from build123d import *

# Parameters (mm, degrees)
SKETCH1_R           = 32.5
BOSS_EXTRUDE1_DEPTH = 230
SKETCH2_R           = 15
BOSS_EXTRUDE2_DEPTH = 100
BOSS_EXTRUDE3_START = 50
SKETCH3_R           = 15
BOSS_EXTRUDE3_DEPTH = 50
BOSS_EXTRUDE4_START = -30
BOSS_EXTRUDE4_DEPTH = 30
SKETCH5_R           = 15
BOSS_EXTRUDE5_DEPTH = 20


with BuildPart() as part:
    # Sketch1 → Boss-Extrude1 (new body)
    with BuildSketch(Plane(origin=(0, 0, 0), x_dir=(1, 0, 0), z_dir=(0, 1, 0))):
        with Locations(Location((0, 0, 0), (0, 0, 270))):
            Circle(SKETCH1_R)
    extrude(amount=BOSS_EXTRUDE1_DEPTH)

    # Sketch2 → Boss-Extrude2 (add)
    with BuildSketch(Plane(origin=(0, 230, 0), x_dir=(1, 0, 0), z_dir=(0, 1, 0))):
        with Locations(Location((0, 0, 0), (0, 0, 270))):
            Circle(SKETCH2_R)
    extrude(amount=BOSS_EXTRUDE2_DEPTH)

    # Sketch3 → Boss-Extrude3 (add)
    with BuildSketch(Plane.XZ.offset(BOSS_EXTRUDE3_START)):
        with Locations(Location((0, 0, 0), (0, 0, 90))):
            Circle(SKETCH3_R)
    extrude(amount=-BOSS_EXTRUDE3_DEPTH)

    # Sketch4 → Boss-Extrude4 (add)
    with BuildSketch(Plane(origin=(0, 330, 0), x_dir=(1, 0, 0), z_dir=(0, 1, 0)).offset(BOSS_EXTRUDE4_START)):
        with BuildLine():
            Line((-3.5, 19.691368668), (-3.5, 14.585952146))
            ThreePointArc((-3.5, 14.585952146), (-5.740251485, 13.858192988), (-7.838951938, 12.788699407))
            Line((-7.838951938, 12.788699407), (-11.449026581, 16.39877405))
            ThreePointArc((-11.449026581, 16.39877405), (-14.142135624, 14.142135624), (-16.39877405, 11.449026581))
            Line((-16.39877405, 11.449026581), (-12.788699407, 7.838951938))
            ThreePointArc((-12.788699407, 7.838951938), (-13.858192988, 5.740251485), (-14.585952146, 3.5))
            Line((-14.585952146, 3.5), (-19.691368668, 3.5))
            ThreePointArc((-19.691368668, 3.5), (-20, 0), (-19.691368668, -3.5))
            Line((-19.691368668, -3.5), (-14.585952146, -3.5))
            ThreePointArc((-14.585952146, -3.5), (-13.858192988, -5.740251485), (-12.788699407, -7.838951938))
            Line((-12.788699407, -7.838951938), (-16.39877405, -11.449026581))
            ThreePointArc((-16.39877405, -11.449026581), (-14.142135624, -14.142135624), (-11.449026581, -16.39877405))
            Line((-11.449026581, -16.39877405), (-7.838951938, -12.788699407))
            ThreePointArc((-7.838951938, -12.788699407), (-5.740251485, -13.858192988), (-3.5, -14.585952146))
            Line((-3.5, -14.585952146), (-3.5, -19.691368668))
            ThreePointArc((-3.5, -19.691368668), (0, -20), (3.5, -19.691368668))
            Line((3.5, -19.691368668), (3.5, -14.585952146))
            ThreePointArc((3.5, -14.585952146), (5.740251485, -13.858192988), (7.838951938, -12.788699407))
            Line((7.838951938, -12.788699407), (11.449026581, -16.39877405))
            ThreePointArc((11.449026581, -16.39877405), (14.142135624, -14.142135624), (16.39877405, -11.449026581))
            Line((16.39877405, -11.449026581), (12.788699407, -7.838951938))
            ThreePointArc((12.788699407, -7.838951938), (13.858192988, -5.740251485), (14.585952146, -3.5))
            Line((14.585952146, -3.5), (19.691368668, -3.5))
            ThreePointArc((19.691368668, -3.5), (20, 0), (19.691368668, 3.5))
            Line((19.691368668, 3.5), (14.585952146, 3.5))
            ThreePointArc((14.585952146, 3.5), (13.858192988, 5.740251485), (12.788699407, 7.838951938))
            Line((12.788699407, 7.838951938), (16.39877405, 11.449026581))
            ThreePointArc((16.39877405, 11.449026581), (14.142135624, 14.142135624), (11.449026581, 16.39877405))
            Line((11.449026581, 16.39877405), (7.838951938, 12.788699407))
            ThreePointArc((7.838951938, 12.788699407), (5.740251485, 13.858192988), (3.5, 14.585952146))
            Line((3.5, 14.585952146), (3.5, 19.691368668))
            ThreePointArc((3.5, 19.691368668), (0, 20), (-3.5, 19.691368668))
        make_face()
    extrude(amount=BOSS_EXTRUDE4_DEPTH)

    # Sketch5 → Boss-Extrude5 (add)
    with BuildSketch(Plane(origin=(0, 330, 0), x_dir=(1, 0, 0), z_dir=(0, 1, 0))):
        with Locations(Location((0, 0, 0), (0, 0, 270))):
            Circle(SKETCH5_R)
    extrude(amount=BOSS_EXTRUDE5_DEPTH)


solid = part.part
Here's how the part is built. I have some questions about the finished solid (model axes, mm). A direction names the side the tool comes from. Round coordinates to 2 decimals unless told otherwise and drop trailing zeros. Loops run counter-clockwise (first coordinate to the right, second up) from the corner with the lowest first, then second, coordinate; pieces in that order, holes last.
1. If I drill on line 1 along Y through (x, z) = (1.5, -25); line 2 along Z through (x, y) = (-29, 132); line 3 along Z through (x, y) = (28.5, 143), over which ranges is the centre line in solid material (lowest first)?
Answer list:
line 1: y = 0 to 230
line 2: z = -14.67 to 14.67
line 3: z = -15.62 to 15.62
2. For P1, Ø2.5, axis at x = 18, z = 1.5, coming from the +Y side; P2, Ø5.5, axis at x = -18.5, y = 311.5, coming from the +Z side; P3, Ø2.5, axis at y = 308, z = -16, coming from the -X side, each with a flat end and sliding along its axis, tell me the tip position at first contact or that it passes through.
Answer list:
P1: stops at y = 330
P2: stops at z = 12.33
P3: stops at x = -13.51
3. If we section it at D-D on z = 28.5: Write out the boundary of the cut face in (x, y), plus the area to 3 significant figures.
Answer list:
outline: (-15.62, 0) - (15.62, 0) - (15.62, 230) - (-15.62, 230) - close
area: 7,190 mm2
4. If we section it at A-A on x = 0: Write out the boundary of the cut face in (y, z), plus the area to 4 significant figures.
Answer list:
outline: (-50, -15) - (0, -15) - (0, -32.5) - (230, -32.5) - (230, -15) - (300, -15) - (300, -20) - (330, -20) - (330, -15) - (350, -15) - (350, 15) - (330, 15) - (330, 20) - (300, 20) - (300, 15) - (230, 15) - (230, 32.5) - (0, 32.5) - (0, 15) - (-50, 15) - close
area: 20,350 mm2
5. We'd pull the mould along Y, two halves only. Please class faces 4 (the face through (12, 300, -12)), 5 (the face through (20, 315, 0)), 6 (the face through (0, 350, 0)): +Y half, -Y half, draft (parallel to the pull), parting line (faces both ways), or undercut.
Answer list:
face 4: undercut
face 5: draft
face 6: +Y half
6. Which directions (+Z, -Z, +X, -X, +Y, -Y) give clear straight access to the entire face, cutting with the end or side of a thin tool? Please do faces 1 (the face through (0, 315, 20)), 2 (the face through (-20, 315, 0)), 3 (the face through (12, 330, 12)).
Answer list:
face 1: +Z, +Y
face 2: -X, +Y
face 3: +Z, +X, +Y
7. If we section it at C-C on y = 20.5: Write out the boundary of the cut face in (x, z).
Answer list:
outline: circle Ø65 at (0, 0)
8. If we section it at B-B on z = 0: Write out the boundary of the cut face in (x, y).
Answer list:
outline: (-32.5, 0) - (-15, 0) - (-15, -50) - (15, -50) - (15, 0) - (32.5, 0) - (32.5, 230) - (15, 230) - (15, 300) - (20, 300) - (20, 330) - (15, 330) - (15, 350) - (-15, 350) - (-15, 330) - (-20, 330) - (-20, 300) - (-15, 300) - (-15, 230) - (-32.5, 230) - close
